Can you work these out from the model? Positions are in its coordinate system, mm. Round coordinates to 2 decimals unless told otherwise and drop trailing zeros. Order: outer loops, then holes, each group sorted by start corner. A loop starts at its lowest first (then second) coordinate and runs counter-clockwise, first axis right, second up.
Q1. If I drill on line 1 (Y direction, x = 0, z = 12); line 2 (X direction, y = -0.5, z = 2); line 3 (Y direction, x = 0, z = 0.1), over which ranges is the centre line in solid material (lowest first)?
Q2. If we section it at C-C (z = 10): Please give me the cut outline in (x, y).
Q3. We'd pull the mould along Y, two halves only. Please class faces 1 (the face through (9, -13, 0.2)), 2 (the face through (0, -20, 0)), 3 (the face through (9, -13, 17.8)), 4 (the face through (22.4, 7.1, 8.9)): pulls with the +Y half, pulls with the -Y half, needs draft (parallel to the pull), parting line crosses it, or undercut.
Q4. Will these pins go through, and if not, where does the flat tip stop? P1, Ø5, axis at x = -4, y = 4.5, coming from the -Z side; P2, Ø1.5, axis at x = 3, z = 7, coming from the -Y side; P3, Ø2, axis at x = -12, y = -9.5, coming from the +Z side; P4, Ø2, axis at x = -15.5, z = 8, coming from the -Y side.
from build123d import *

# Parameters (mm, degrees)
SKETCH_1_R          = 23.5
SKETCH_1_R_2        = 10
EXTRUDE_1_DEPTH     = 18
FILLET_1_R          = 1
SKETCH_2_R          = 19.75
SKETCH_2_R_2        = 14.15
CUT_EXTRUDE_1_DEPTH = 0.2
CUT_EXTRUDE_START   = -17.8
SKETCH_2_3_R        = 19.75
SKETCH_2_3_R_2      = 14.15
CUT_EXTRUDE_2_DEPTH = 0.2


with BuildPart() as part:
    # Эскиз1 → Бобышка-Вытянуть1 (new body)
    with BuildSketch(Plane.XY):
        Circle(SKETCH_1_R)
        Circle(SKETCH_1_R_2, mode=Mode.SUBTRACT)
    extrude(amount=EXTRUDE_1_DEPTH)

    # Скругление1
    fillet_1_edges = [part.edges().sort_by_distance(p)[0] for p in [
        (-23.5, 0, 0),
        (-23.5, 0, 18),
        (-10, 0, 0),
        (-10, 0, 18),
    ]]
    fillet(fillet_1_edges, radius=FILLET_1_R)

    # Эскиз2 → Вырез-Вытянуть1 (cut)
    with BuildSketch(Plane.XY.offset(18)):
        Circle(SKETCH_2_R)
        Circle(SKETCH_2_R_2, mode=Mode.SUBTRACT)
    extrude(amount=-CUT_EXTRUDE_1_DEPTH, mode=Mode.SUBTRACT)

    # Эскиз2<3> → Вырез-Вытянуть2 (cut)
    with BuildSketch(Plane.XY.offset(18).offset(CUT_EXTRUDE_START)):
        Circle(SKETCH_2_3_R)
        Circle(SKETCH_2_3_R_2, mode=Mode.SUBTRACT)
    extrude(amount=-CUT_EXTRUDE_2_DEPTH, mode=Mode.SUBTRACT)


solid = part.part
Solution:
1. line 1: y = -23.5 to -10, 10 to 23.5
1. line 2: x = -23.49 to -9.99, 9.99 to 23.49
1. line 3: y = -22.94 to -19.75, -14.15 to -10.56, 10.56 to 14.15, 19.75 to 22.94
2. outline: circle Ø47 at (0, 0); hole circle Ø20 at (0, 0)
3. face 1: undercut
3. face 2: needs draft
3. face 3: undercut
3. face 4: parting line crosses it
4. P1: passes through
4. P2: stops at y = -23.39
4. P3: stops at z = 17.8
4. P4: stops at y = -18.49
